Check sheet for the drawn part. Datum: minimum x, y, z corner. Units: mm. A direction names the side the tool comes from. Round coordinates to 2 decimals unless told otherwise and drop trailing zeros. Write each loop counter-clockwise with the first axis right and the second up, starting at its lowest first coordinate (ties: lowest second). Pieces come first, ordered by that corner, then holes. Notation, with made-up numbers: M -25,60 L 23,60 A22 ccw 23,67 Z; hole C 68.25,0 d1. An arc over 180 degrees is marked long. Put each result on its own line as item: value.
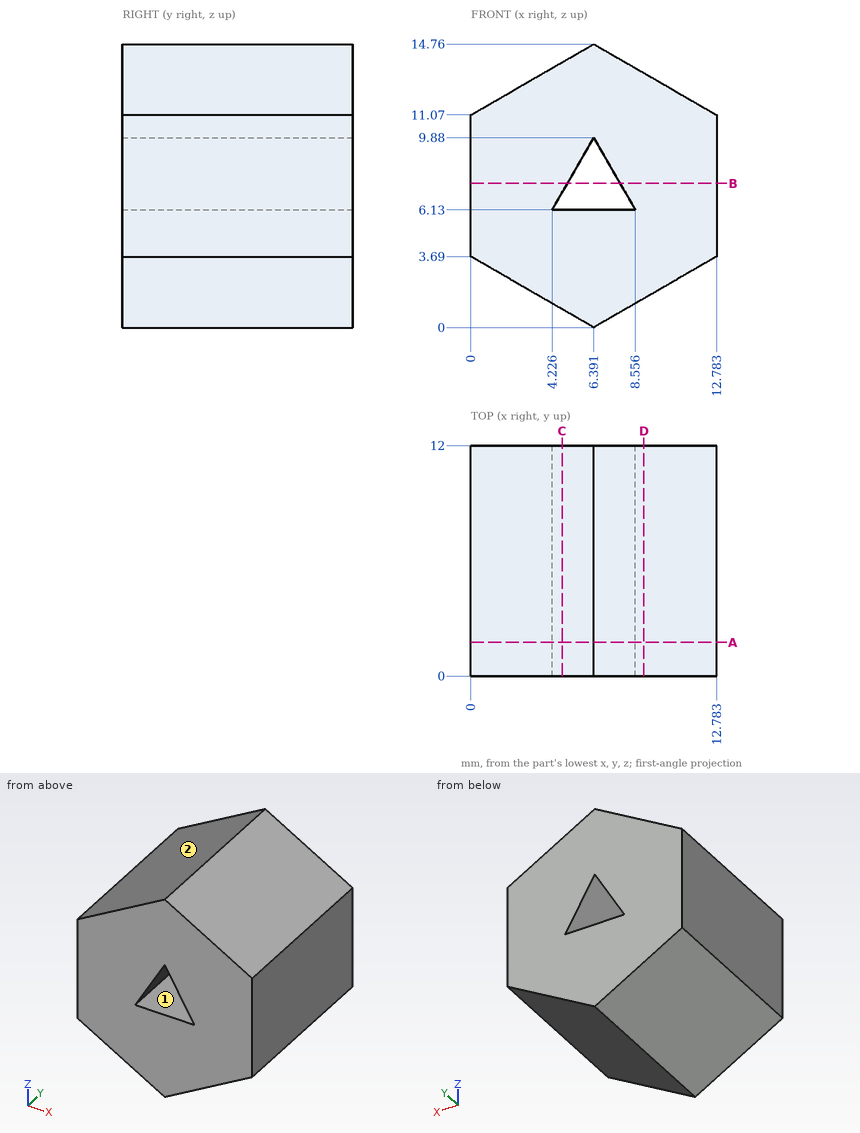
1. Cross-section at A-A (y = 1.75). Enter the section's corners in (x, z).
Computed values:
outline: M 0,3.69 L 6.39,0 L 12.78,3.69 L 12.78,11.07 L 6.39,14.76 L 0,11.07 Z; hole M 4.23,6.13 L 8.56,6.13 L 6.39,9.88 Z
2. Depth check by flat-ended pin: pin 1 Ø6 at (x, y) = (9, 6.5) entering from +Z; pin 2 Ø1.3 at (x, y) = (7.5, 4.5) entering from +Z (1 decimal); pin 3 Ø2 at (x, y) = (10.5, 7.5) entering from -Z (1 decimal). Enter the tip coordinate at first touch or a pass-through.
Computed values:
pin 1: stops at z = 14.76
pin 2: stops at z = 14.5
pin 3: stops at z = 1.8
3. Cross-section at D-D (x = 9). Enter the section's corners in (y, z), then the cut area to 3 significant figures.
Computed values:
outline: M 0,1.51 L 12,1.51 L 12,13.25 L 0,13.25 Z
area: 141 mm2
4. Access from +Z, -Z, +X, -X, +Y, -Y to the whole of each face (thin tool, end or side, straight path). Record for the marked faces 1 and 2.
Computed values:
face 1: +Y, -Y
face 2: +Z, -X, +Y, -Y
5. Cross-section at B-B (z = 7.5). Enter the section's corners in (x, y) (1 decimal).
Computed values:
outline: M 0,0 L 5,0 L 5,12 L 0,12 Z; M 7.8,0 L 12.8,0 L 12.8,12 L 7.8,12 Z
6. Scan lines: probe 1 along Z at (x, y) = (6, 1) (1 decimal); probe 2 along Z at (x, y) = (4.5, 1.25) (1 decimal); probe 3 along X at (y, z) = (2.75, 7) (1 decimal). Record each from-to range of solid material in increasing order.
Computed values:
probe 1: z = 0.2 to 6.1, 9.2 to 14.5
probe 2: z = 1.1 to 6.1, 6.6 to 13.7
probe 3: x = 0 to 4.7, 8.1 to 12.8
7. Cross-section at C-C (x = 4.75). Enter the section's corners in (y, z).
Computed values:
outline: M 0,0.95 L 12,0.95 L 12,6.13 L 0,6.13 Z; M 0,7.04 L 12,7.04 L 12,13.81 L 0,13.81 Z
